CAD build for the part. Positions are in the model's coordinates, mm. Give positions to 0.01 mm unless a question says otherwise; leave off trailing zeros. Order: outer loops, then holes, each group sorted by start corner. A loop starts at its lowest first (then second) coordinate and runs counter-clockwise, first axis right, second up. Notation, with made-up numbers: M 60.5,-5 L 74.5,-5 A13 cw 74.5,13 Z; hole C -30.5,36 d10. An arc over 180 degrees is marked long. Put each result on its own line as item: value. Start each with the question number.
1) Drill centre lines: line 1 (X direction, y = 2.5, z = -176); line 2 (X direction, y = 1.55, z = -118); line 3 (X direction, y = -1.45, z = -134). Where is each one in solid material? Low to high. Write a range as [from, to].
2) Pin check, flat tips, straight feed: pin 1 (2 mm diameter, centred on x = 58, y = 1.5, fed in from +Z); pin 2 (3 mm diameter, centred on y = -1, z = -79, fed in from +X); pin 3 (3 mm diameter, centred on y = -0.5, z = -78, fed in from -X); pin 4 (3.5 mm diameter, centred on x = 110.06, z = -113.02, fed in from +Y). Stop position of each tip, or through.
3) Cut at C-C (z = -21). Write the cut outline in (x, y).
4) Cut at A-A (x = 254). Write the cut outline in (y, z), and give its area (3 significant figures).
5) Cut at B-B (y = -0.8). Give the number of separate pieces and of enclosed holes in the cut face, and give its area (3 significant figures).
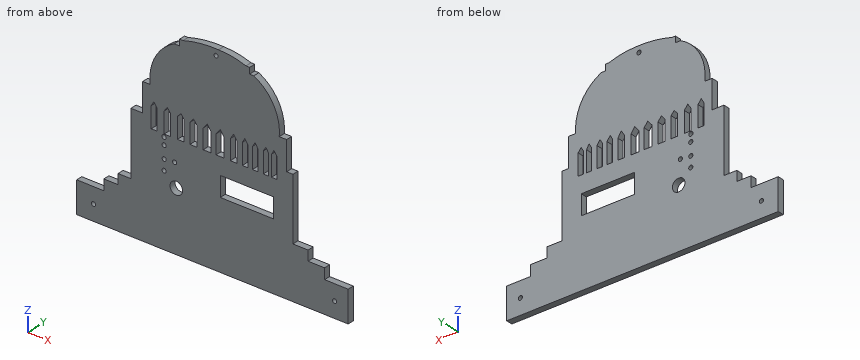
```python
from build123d import *

# Parameters (mm, degrees)
F0_R          = 2
F0_R_2        = 6
F0_W          = 51
F0_H          = 19
F1_DEPTH      = 3
F1_DEPTH_BACK = 3
F2_DEPTH      = 3


with BuildPart() as f1:
    # F0 (on Front) → F1 (new body, two sides)
    with BuildSketch(Plane.XZ) as f1_sk:
        Polygon((52.472187, -161.24922), (26.581464, -161.24922), (26.581464, -191.24922), (285.798032, -191.24922), (285.798032, -161.24922), (263.240432, -161.24922), align=None)
        with Locations((42.581464, -176.24922)):
            Circle(F0_R, mode=Mode.SUBTRACT)
        with Locations((272.798032, -176.24922)):
            Circle(F0_R, mode=Mode.SUBTRACT)
        Polygon((52.472187, -151.052892), (52.472187, -161.24922), (263.240432, -161.24922), (263.240432, -151.052892), (247.487148, -151.052892), (66.052614, -151.052892), align=None)
        Polygon((66.052614, -141.450859), (66.052614, -151.052892), (247.487148, -151.052892), (247.487148, -141.450859), (233.003996, -141.450859), (78.357242, -141.450859), align=None)
        Polygon((78.357242, -80.774188), (78.357242, -141.450859), (233.003996, -141.450859), (233.003996, -81.450859), (226.991639, -81.450859), (221.457498, -91.450859), (217.57254, -91.450859), (212.587059, -91.450859), (209.57654, -91.450859), (204.673612, -91.450859), (199.559822, -91.450859), (194.298849, -91.450859), (190.03109, -91.450859), (184.636118, -91.450859), (179.739267, -91.450859), (173.225334, -91.450859), (167.207984, -91.450859), (159.590964, -91.450859), (154.603716, -91.450859), (147.321078, -91.450859), (141.375312, -91.450859), (134.690078, -91.450859), (128.813708, -91.450859), (122.717327, -91.450859), (116.260559, -91.450859), (110.056117, -91.450859), (103.166793, -91.450859), (97.665451, -91.450859), (89.594654, -80.774188), align=None)
        with Locations((121.645503, -133.909166)):
            Circle(F0_R_2, mode=Mode.SUBTRACT)
        with Locations((110.056117, -123.021676)):
            Circle(F0_R, mode=Mode.SUBTRACT)
        with Locations((110.056117, -113.021676)):
            Circle(F0_R, mode=Mode.SUBTRACT)
        with Locations((120.015055, -112.116382)):
            Circle(F0_R, mode=Mode.SUBTRACT)
        with Locations((110.056117, -101.021676)):
            Circle(F0_R, mode=Mode.SUBTRACT)
        with Locations((189.145503, -117.110979)):
            Rectangle(F0_W, F0_H, mode=Mode.SUBTRACT)
        with Locations((109.930342, -94.096712)):
            Circle(F0_R, mode=Mode.SUBTRACT)
        Polygon((89.594654, -53.617763), (89.594654, -80.774188), (97.665451, -91.450859), (97.665451, -71.488872), (100.125542, -67.256524), (103.166793, -71.279724), (103.166793, -91.450859), (110.056117, -91.450859), (110.056117, -71.586892), (112.953584, -67.329317), (116.260559, -71.586892), (116.260559, -91.450859), (122.717327, -91.450859), (122.717327, -71.556566), (126.055585, -68.058384), (128.813708, -71.556566), (128.813708, -91.450859), (134.690078, -91.450859), (134.690078, -72.430915), (138.060334, -68.216196), (141.375312, -72.430915), (141.375312, -91.450859), (147.321078, -91.450859), (147.321078, -72.639709), (151.104841, -67.914439), (154.603716, -72.639709), (154.603716, -91.450859), (159.590964, -91.450859), (159.590964, -73.276494), (163.56732, -68.100847), (167.207984, -73.276494), (167.207984, -91.450859), (173.225334, -91.450859), (173.225334, -72.414774), (176.386258, -67.362841), (179.739267, -72.414774), (179.739267, -91.450859), (184.636118, -91.450859), (184.636118, -71.586892), (186.982751, -67.329317), (190.03109, -71.586892), (190.03109, -91.450859), (194.298849, -91.450859), (194.298849, -71.586892), (196.836814, -67.257442), (199.559822, -71.586892), (199.559822, -91.450859), (204.673612, -91.450859), (204.673612, -71.586892), (207.251813, -67.329317), (209.57654, -71.586892), (209.57654, -91.450859), (212.587059, -91.450859), (212.587059, -71.512245), (214.826435, -67.556024), (217.57254, -71.284115), (217.57254, -91.450859), (221.457498, -91.450859), (226.991639, -81.450859), (226.991639, -53.721661), (219.91986, -53.783055), (198.035091, -53.973049), (96.72894, -53.617763), align=None)
        with BuildLine():
            ThreePointArc((119.692937, -10.181499), (101.370795, -28.283366), (96.72894, -53.617763))
            Line((96.72894, -53.617763), (198.035091, -53.973049))
            Line((198.035091, -53.973049), (219.91986, -53.783055))
            ThreePointArc((219.91986, -53.783055), (214.480878, -28.243005), (195.621964, -10.181499))
            Line((195.621964, -10.181499), (191.704065, -10.181499))
            Line((191.704065, -10.181499), (191.704065, -4.340463))
            Line((191.704065, -4.340463), (188.154012, -4.340463))
            ThreePointArc((188.154012, -4.340463), (175.263432, -1.007217), (161.987022, 0))
            ThreePointArc((161.987022, 0), (144.870074, -0.788162), (128.10725, -4.340463))
            Line((128.10725, -4.340463), (124.78289, -4.340463))
            Line((124.78289, -4.340463), (124.78289, -10.181499))
            Line((124.78289, -10.181499), (119.692937, -10.181499))
        make_face()
        with Locations((159.579262, -5.946493)):
            Circle(F0_R, mode=Mode.SUBTRACT)
    extrude(amount=F1_DEPTH)
    extrude(f1_sk.sketch, amount=-F1_DEPTH_BACK)

    # F0 (on Front) → F2 (join)
    with BuildSketch(Plane.XZ):
        Polygon((52.472187, -161.24922), (26.581464, -161.24922), (26.581464, -191.24922), (285.798032, -191.24922), (285.798032, -161.24922), (263.240432, -161.24922), align=None)
        with Locations((42.581464, -176.24922)):
            Circle(F0_R, mode=Mode.SUBTRACT)
        with Locations((272.798032, -176.24922)):
            Circle(F0_R, mode=Mode.SUBTRACT)
        Polygon((52.472187, -151.052892), (52.472187, -161.24922), (263.240432, -161.24922), (263.240432, -151.052892), (247.487148, -151.052892), (66.052614, -151.052892), align=None)
        Polygon((66.052614, -141.450859), (66.052614, -151.052892), (247.487148, -151.052892), (247.487148, -141.450859), (233.003996, -141.450859), (78.357242, -141.450859), align=None)
        Polygon((78.357242, -80.774188), (78.357242, -141.450859), (233.003996, -141.450859), (233.003996, -81.450859), (226.991639, -81.450859), (221.457498, -91.450859), (217.57254, -91.450859), (212.587059, -91.450859), (209.57654, -91.450859), (204.673612, -91.450859), (199.559822, -91.450859), (194.298849, -91.450859), (190.03109, -91.450859), (184.636118, -91.450859), (179.739267, -91.450859), (173.225334, -91.450859), (167.207984, -91.450859), (159.590964, -91.450859), (154.603716, -91.450859), (147.321078, -91.450859), (141.375312, -91.450859), (134.690078, -91.450859), (128.813708, -91.450859), (122.717327, -91.450859), (116.260559, -91.450859), (110.056117, -91.450859), (103.166793, -91.450859), (97.665451, -91.450859), (89.594654, -80.774188), align=None)
        with Locations((121.645503, -133.909166)):
            Circle(F0_R_2, mode=Mode.SUBTRACT)
        with Locations((110.056117, -123.021676)):
            Circle(F0_R, mode=Mode.SUBTRACT)
        with Locations((110.056117, -113.021676)):
            Circle(F0_R, mode=Mode.SUBTRACT)
        with Locations((120.015055, -112.116382)):
            Circle(F0_R, mode=Mode.SUBTRACT)
        with Locations((110.056117, -101.021676)):
            Circle(F0_R, mode=Mode.SUBTRACT)
        with Locations((189.145503, -117.110979)):
            Rectangle(F0_W, F0_H, mode=Mode.SUBTRACT)
        with Locations((109.930342, -94.096712)):
            Circle(F0_R, mode=Mode.SUBTRACT)
        Polygon((89.594654, -53.617763), (89.594654, -80.774188), (97.665451, -91.450859), (97.665451, -71.488872), (100.125542, -67.256524), (103.166793, -71.279724), (103.166793, -91.450859), (110.056117, -91.450859), (110.056117, -71.586892), (112.953584, -67.329317), (116.260559, -71.586892), (116.260559, -91.450859), (122.717327, -91.450859), (122.717327, -71.556566), (126.055585, -68.058384), (128.813708, -71.556566), (128.813708, -91.450859), (134.690078, -91.450859), (134.690078, -72.430915), (138.060334, -68.216196), (141.375312, -72.430915), (141.375312, -91.450859), (147.321078, -91.450859), (147.321078, -72.639709), (151.104841, -67.914439), (154.603716, -72.639709), (154.603716, -91.450859), (159.590964, -91.450859), (159.590964, -73.276494), (163.56732, -68.100847), (167.207984, -73.276494), (167.207984, -91.450859), (173.225334, -91.450859), (173.225334, -72.414774), (176.386258, -67.362841), (179.739267, -72.414774), (179.739267, -91.450859), (184.636118, -91.450859), (184.636118, -71.586892), (186.982751, -67.329317), (190.03109, -71.586892), (190.03109, -91.450859), (194.298849, -91.450859), (194.298849, -71.586892), (196.836814, -67.257442), (199.559822, -71.586892), (199.559822, -91.450859), (204.673612, -91.450859), (204.673612, -71.586892), (207.251813, -67.329317), (209.57654, -71.586892), (209.57654, -91.450859), (212.587059, -91.450859), (212.587059, -71.512245), (214.826435, -67.556024), (217.57254, -71.284115), (217.57254, -91.450859), (221.457498, -91.450859), (226.991639, -81.450859), (226.991639, -53.721661), (219.91986, -53.783055), (198.035091, -53.973049), (96.72894, -53.617763), align=None)
        with BuildLine():
            ThreePointArc((119.692937, -10.181499), (101.370795, -28.283366), (96.72894, -53.617763))
            Line((96.72894, -53.617763), (198.035091, -53.973049))
            Line((198.035091, -53.973049), (219.91986, -53.783055))
            ThreePointArc((219.91986, -53.783055), (214.480878, -28.243005), (195.621964, -10.181499))
            Line((195.621964, -10.181499), (191.704065, -10.181499))
            Line((191.704065, -10.181499), (191.704065, -4.340463))
            Line((191.704065, -4.340463), (188.154012, -4.340463))
            ThreePointArc((188.154012, -4.340463), (175.263432, -1.007217), (161.987022, 0))
            ThreePointArc((161.987022, 0), (144.870074, -0.788162), (128.10725, -4.340463))
            Line((128.10725, -4.340463), (124.78289, -4.340463))
            Line((124.78289, -4.340463), (124.78289, -10.181499))
            Line((124.78289, -10.181499), (119.692937, -10.181499))
        make_face()
        with Locations((159.579262, -5.946493)):
            Circle(F0_R, mode=Mode.SUBTRACT)
    extrude(amount=F2_DEPTH)


solid = f1.part
```
Solution:
1. line 1: [26.58, 40.6], [44.57, 270.81], [274.78, 285.8]
1. line 2: [78.36, 163.65], [214.65, 233]
1. line 3: [78.36, 115.65], [127.64, 233]
2. pin 1: z = -151.05
2. pin 2: x = 226.99
2. pin 3: x = 89.59
2. pin 4: through
3. outline: M 106.23,-3 L 209.44,-3 L 209.44,3 L 106.23,3 Z
4. outline: M -3,-191.25 L 3,-191.25 L 3,-151.05 L -3,-151.05 Z
4. area: 241 mm²
5. separate pieces: 1
5. enclosed holes: 21
5. area: 27,600 mm²
